The listing builds one solid part. Answer for the finished solid, in the listing's coordinates (mm). A direction names the side the tool comes from. Coordinates: 2 decimals unless noted, no trailing zeros. Write each loop counter-clockwise with the first axis right and the second up, starting at its lowest first coordinate (ties: lowest second). Pieces come first, ordered by that corner, then holes.
from build123d import *

# Parameters (mm, degrees)
EXTRUDE_THIN1_DEPTH = 304.8
SKETCH2_W           = 69.85
SKETCH2_H           = 88.9
CUT_EXTRUDE1_DEPTH  = 324.85
SKETCH3_W           = 533.4
SKETCH3_H           = 44.45
CUT_EXTRUDE2_DEPTH  = 4.175


with BuildPart() as part:
    # Sketch1 → Extrude-Thin1 (new body)
    with BuildSketch(Plane(origin=(0, 0, 0), x_dir=(1, 0, 0), z_dir=(0, 1, 0))):
        Polygon((-349.25, 196.85), (-349.25, -127), (-101.6, -127), (292.1, -127), (349.25, -127), (349.25, 196.85), (346.075, 196.85), (346.075, -123.825), (292.1, -123.825), (-101.6, -123.825), (-346.075, -123.825), (-346.075, 196.85), align=None)
    extrude(amount=EXTRUDE_THIN1_DEPTH)

    # Sketch2 → Cut-Extrude1 (cut, through all)
    with BuildSketch(Plane(origin=(-139.504532993, -186.632694872, 127), x_dir=(1, 0, 0), z_dir=(0, 0, 1))):
        with Locations((-171.645467007, 231.082694872)):
            Rectangle(SKETCH2_W, SKETCH2_H)
    extrude(amount=-CUT_EXTRUDE1_DEPTH, mode=Mode.SUBTRACT)

    # Sketch3 → Cut-Extrude2 (cut, through all)
    with BuildSketch(Plane(origin=(0, 0, 123.825), x_dir=(-1, 0, 0), z_dir=(0, 0, -1))):
        with Locations((9.525, 22.225)):
            Rectangle(SKETCH3_W, SKETCH3_H)
    extrude(amount=-CUT_EXTRUDE2_DEPTH, mode=Mode.SUBTRACT)


solid = part.part
1. Section B-B on z = -161 is taken. Give the vertices of the cut face in (x, y) (3 decimals).
Results found:
outline: (-349.25, 0) - (-346.075, 0) - (-346.075, 304.8) - (-349.25, 304.8) - close; (346.075, 0) - (349.25, 0) - (349.25, 304.8) - (346.075, 304.8) - close
2. Find the intervals of material crossed by L1, parallel to X at y = 113, z = -167 (3 decimals); L2, parallel to Z at x = -230, y = 276.5 (3 decimals), in increasing order.
Results found:
L1: x = -349.25 to -346.075, 346.075 to 349.25
L2: z = 123.825 to 127
3. Section A-A on y = 59.5 is taken. Give the vertices of the cut face in (x, z) (3 decimals).
Results found:
outline: (-349.25, -196.85) - (-346.075, -196.85) - (-346.075, 127) - (-349.25, 127) - close; (-276.225, 123.825) - (346.075, 123.825) - (346.075, -196.85) - (349.25, -196.85) - (349.25, 127) - (-276.225, 127) - close
4. Flat-ended cylindrical pins translate along their axes: P1, Ø1.6, axis at x = -45, z = 125, coming from the -Y side; P2, Ø2, axis at x = 171, y = 181, coming from the -Z side (3 decimals); P3, Ø1, axis at x = -299, z = 126, coming from the -Y side. Find the tip coordinate at first contact, or state that the pin passes through.
Results found:
P1: stops at y = 44.45
P2: stops at z = 123.825
P3: stops at y = 88.9
5. Section C-C on y = 180 is taken. Give the vertices of the cut face in (x, z) (3 decimals), then the cut area to 3 significant figures.
Results found:
outline: (-349.25, -196.85) - (-346.075, -196.85) - (-346.075, 123.825) - (346.075, 123.825) - (346.075, -196.85) - (349.25, -196.85) - (349.25, 127) - (-349.25, 127) - close
area: 4,250 mm2
6. Section D-D on x = 26.5 is taken. Give the vertices of the cut face in (y, z) (3 decimals).
Results found:
outline: (44.45, 123.825) - (304.8, 123.825) - (304.8, 127) - (44.45, 127) - close
7. For a pull along X with two mould halves and no side action, classify faces 1 (the flat face through (-5, 184, 127)), 2 (the flat face through (349.25, 150, -33)), 3 (the flat face through (5, 184, 123.825)), 4 (the flat face through (-349.25, 150, -37)) as pulls with the +X half, pulls with the -X half, needs draft (parallel to the pull), parting line crosses it, or undercut.
Results found:
face 1: needs draft
face 2: pulls with the +X half
face 3: undercut
face 4: pulls with the -X half
8. A tool of negligible diameter and unlimited length cuts with its end or side. For faces 5 (the flat face through (347, 0, -36)), 6 (the flat face through (346.075, 150, -39)), from which of +Z, -Z, +X, -X, +Y, -Y can it reach the whole face along a straight path? Write none if from no direction.
Results found:
face 5: +Z, -Z, +X, -X, -Y
face 6: -Z, +Y, -Y
